```python
from build123d import *

# Parameters (mm, degrees)
SKETCH_1_R          = 3.75
SKETCH_1_R_2        = 2.75
EXTRUDE_436_DEPTH   = 4
EXTRUDE_START       = 4
SKETCH_2_R          = 1.7
SKETCH_2_R_2        = 2.75
EXTRUDE_712_DEPTH   = 5
SKETCH_3_R          = 2.9
EXTRUDE_5_8_DEPTH   = 9
SKETCH_4_R          = 2.9
EXTRUDE_5_8_2_DEPTH = 9


with BuildPart() as part:
    # 草图1 → Extrude 436 (new body)
    with BuildSketch(Plane.XY):
        Polygon((-44.899888641, -10), (-44.2082264, -12.713485699), (-43.352738806, -15.379858192), (-42.336596099, -17.989236526), (-41.163563864, -20.531950955), (-39.837989085, -22.998578775), (-38.364784033, -25.379979238), (-36.74940806, -27.667327432), (-34.997847373, -29.852146979), (-33.116592846, -31.926341448), (-31.112615968, -33.882224361), (-28.993343009, -35.712547671), (-26.7666275, -37.410528629), (-24.440721127, -38.969874914), (-22.024243155, -40.384807953), (-19.526148488, -41.650084336), (-16.955694479, -42.761015244), (-14.322406631, -43.713483827), (-11.636043292, -44.503960459), (-8.906559497, -45.129515818), (-6.144070075, -45.587831742), (-3.358812166, -45.87720982), (-0.561107284, -45.996577684), (2.238676931, -45.945492985), (5.030165132, -45.72414503), (7.803012717, -45.333354084), (10.546944161, -44.774568327), (13.251791096, -44.049858487), (15.907529991, -43.161910171), (18.504319299, -42.114013906), (21.032535927, -40.910052952), (23.482810893, -39.554488905), (25.846064052, -38.052345171), (28.11353774, -36.409188342), (30.276829231, -34.631107573), (32.327921871, -32.724692016), (34.25921479, -30.697006401), (36.063551069, -28.555564857), (37.734244259, -26.308303066), (39.265103162, -23.963548854), (40.650454772, -21.529991333), (41.885165301, -19.016648698), (42.9646592, -16.432834808), (43.884936117, -13.788124675), (44.64258572, -11.092318975), (45.234800338, -8.355407734), (45.659385361, -5.587533306), (45.914767377, -2.798952785), (46, 0), (45.914767377, 2.798952785), (45.659385361, 5.587533306), (45.234800338, 8.355407734), (44.64258572, 11.092318975), (43.884936117, 13.788124675), (42.9646592, 16.432834808), (41.885165301, 19.016648698), (40.650454772, 21.529991333), (39.265103162, 23.963548854), (37.734244259, 26.308303066), (36.063551069, 28.555564857), (34.25921479, 30.697006401), (32.327921871, 32.724692016), (30.276829231, 34.631107573), (28.11353774, 36.409188342), (25.846064052, 38.052345171), (23.482810893, 39.554488905), (21.032535927, 40.910052952), (18.504319299, 42.114013906), (15.907529991, 43.161910171), (13.251791096, 44.049858487), (10.546944161, 44.774568327), (7.803012717, 45.333354084), (5.030165132, 45.72414503), (2.238676931, 45.945492985), (-0.561107284, 45.996577684), (-3.358812166, 45.87720982), (-6.144070075, 45.587831742), (-8.906559497, 45.129515818), (-11.636043292, 44.503960459), (-14.322406631, 43.713483827), (-16.955694479, 42.761015244), (-19.526148488, 41.650084336), (-22.024243155, 40.384807953), (-24.440721127, 38.969874914), (-26.7666275, 37.410528629), (-28.993343009, 35.712547671), (-31.112615968, 33.882224361), (-33.116592846, 31.926341448), (-34.997847373, 29.852146979), (-36.74940806, 27.667327432), (-38.364784033, 25.379979238), (-39.837989085, 22.998578775), (-41.163563864, 20.531950955), (-42.336596099, 17.989236526), (-43.352738806, 15.379858192), (-44.2082264, 12.713485699), (-44.899888641, 10), (12, 10), (12, -10), align=None)
        with Locations((-14.845, -14.845)):
            Circle(SKETCH_1_R, mode=Mode.SUBTRACT)
        with Locations((-14.845, 14.845)):
            Circle(SKETCH_1_R, mode=Mode.SUBTRACT)
        with Locations((14.845, -14.845)):
            Circle(SKETCH_1_R, mode=Mode.SUBTRACT)
        with Locations((14.845, 14.845)):
            Circle(SKETCH_1_R, mode=Mode.SUBTRACT)
        with Locations((0, -40.5)):
            Circle(SKETCH_1_R_2, mode=Mode.SUBTRACT)
        with Locations((0, 40.5)):
            Circle(SKETCH_1_R_2, mode=Mode.SUBTRACT)
        with Locations((40.5, 0)):
            Circle(SKETCH_1_R_2, mode=Mode.SUBTRACT)
    extrude(amount=EXTRUDE_436_DEPTH)

    # 草图2 → Extrude 712 (add)
    with BuildSketch(Plane.XY.offset(EXTRUDE_START)):
        Polygon((-44.899888641, -10), (-44.2082264, -12.713485699), (-43.352738806, -15.379858192), (-42.336596099, -17.989236526), (-41.163563864, -20.531950955), (-39.837989085, -22.998578775), (-38.364784033, -25.379979238), (-36.74940806, -27.667327432), (-34.997847373, -29.852146979), (-33.116592846, -31.926341448), (-31.112615968, -33.882224361), (-28.993343009, -35.712547671), (-26.7666275, -37.410528629), (-24.440721127, -38.969874914), (-22.024243155, -40.384807953), (-19.526148488, -41.650084336), (-16.955694479, -42.761015244), (-14.322406631, -43.713483827), (-11.636043292, -44.503960459), (-8.906559497, -45.129515818), (-6.144070075, -45.587831742), (-3.358812166, -45.87720982), (-0.561107284, -45.996577684), (2.238676931, -45.945492985), (5.030165132, -45.72414503), (7.803012717, -45.333354084), (10.546944161, -44.774568327), (13.251791096, -44.049858487), (15.907529991, -43.161910171), (18.504319299, -42.114013906), (21.032535927, -40.910052952), (23.482810893, -39.554488905), (25.846064052, -38.052345171), (28.11353774, -36.409188342), (30.276829231, -34.631107573), (32.327921871, -32.724692016), (34.25921479, -30.697006401), (36.063551069, -28.555564857), (37.734244259, -26.308303066), (39.265103162, -23.963548854), (40.650454772, -21.529991333), (41.885165301, -19.016648698), (42.9646592, -16.432834808), (43.884936117, -13.788124675), (44.64258572, -11.092318975), (45.234800338, -8.355407734), (45.659385361, -5.587533306), (45.914767377, -2.798952785), (46, 0), (45.914767377, 2.798952785), (45.659385361, 5.587533306), (45.234800338, 8.355407734), (44.64258572, 11.092318975), (43.884936117, 13.788124675), (42.9646592, 16.432834808), (41.885165301, 19.016648698), (40.650454772, 21.529991333), (39.265103162, 23.963548854), (37.734244259, 26.308303066), (36.063551069, 28.555564857), (34.25921479, 30.697006401), (32.327921871, 32.724692016), (30.276829231, 34.631107573), (28.11353774, 36.409188342), (25.846064052, 38.052345171), (23.482810893, 39.554488905), (21.032535927, 40.910052952), (18.504319299, 42.114013906), (15.907529991, 43.161910171), (13.251791096, 44.049858487), (10.546944161, 44.774568327), (7.803012717, 45.333354084), (5.030165132, 45.72414503), (2.238676931, 45.945492985), (-0.561107284, 45.996577684), (-3.358812166, 45.87720982), (-6.144070075, 45.587831742), (-8.906559497, 45.129515818), (-11.636043292, 44.503960459), (-14.322406631, 43.713483827), (-16.955694479, 42.761015244), (-19.526148488, 41.650084336), (-22.024243155, 40.384807953), (-24.440721127, 38.969874914), (-26.7666275, 37.410528629), (-28.993343009, 35.712547671), (-31.112615968, 33.882224361), (-33.116592846, 31.926341448), (-34.997847373, 29.852146979), (-36.74940806, 27.667327432), (-38.364784033, 25.379979238), (-39.837989085, 22.998578775), (-41.163563864, 20.531950955), (-42.336596099, 17.989236526), (-43.352738806, 15.379858192), (-44.2082264, 12.713485699), (-44.899888641, 10), (12, 10), (12, -10), align=None)
        with Locations((-14.845, -14.845)):
            Circle(SKETCH_2_R, mode=Mode.SUBTRACT)
        with Locations((-14.845, 14.845)):
            Circle(SKETCH_2_R, mode=Mode.SUBTRACT)
        with Locations((14.845, -14.845)):
            Circle(SKETCH_2_R, mode=Mode.SUBTRACT)
        with Locations((14.845, 14.845)):
            Circle(SKETCH_2_R, mode=Mode.SUBTRACT)
        with Locations((0, -40.5)):
            Circle(SKETCH_2_R_2, mode=Mode.SUBTRACT)
        with Locations((0, 40.5)):
            Circle(SKETCH_2_R_2, mode=Mode.SUBTRACT)
        with Locations((40.5, 0)):
            Circle(SKETCH_2_R_2, mode=Mode.SUBTRACT)
    extrude(amount=EXTRUDE_712_DEPTH)

    # 草图3 → Extrude 5.8 (add)
    with BuildSketch(Plane.XY):
        with BuildLine():
            Line((-33.234018716, -14.849242405), (-69.028961031, -56.301038969))
            ThreePointArc((-69.028961031, -56.301038969), (-69.028961031, -69.028961031), (-56.301038969, -69.028961031))
            Line((-56.301038969, -69.028961031), (-14.849242405, -33.234018716))
            Line((-14.849242405, -33.234018716), (-33.234018716, -14.849242405))
        make_face()
        with Locations((-62.665, -62.665)):
            Circle(SKETCH_3_R, mode=Mode.SUBTRACT)
    extrude(amount=EXTRUDE_5_8_DEPTH)

    # 草图4 → Extrude 5.8 2 (add)
    with BuildSketch(Plane.XY):
        with BuildLine():
            Line((-14.849242405, 33.234018716), (-56.301038969, 69.028961031))
            ThreePointArc((-56.301038969, 69.028961031), (-69.028961031, 69.028961031), (-69.028961031, 56.301038969))
            Line((-69.028961031, 56.301038969), (-33.234018716, 14.849242405))
            Line((-33.234018716, 14.849242405), (-14.849242405, 33.234018716))
        make_face()
        with Locations((-62.665, 62.665)):
            Circle(SKETCH_4_R, mode=Mode.SUBTRACT)
    extrude(amount=EXTRUDE_5_8_2_DEPTH)


solid = part.part
```
Check sheet for the modelled part. Datum: model origin and axes. Units: mm. A direction names the side the tool comes from. Give positions to 0.01 mm unless a question says otherwise; leave off trailing zeros. Order: outer loops, then holes, each group sorted by start corner. A loop starts at its lowest first (then second) coordinate and runs counter-clockwise, first axis right, second up. Notation, with made-up numbers: M 54.25,-31.5 L 60.25,-31.5 A23 ccw 60.25,-22.5 Z; hole C 84,2 d2. An arc over 180 degrees is marked long. Answer in a Markdown table with one row per item. Add a question column.
Q1. Release check for a two-part mould opening along X. For faces 1 (the flat face through (13, -15, 4)), 2 (the cylindrical face through (-68.887, 69.167, 4.437)), 3 (the flat face through (45.79, 4.17, 4.44)), 4 (the flat face through (16, 13, 4)) record: released by +X, released by -X, zero draft, split by the parting line, or undercut.
Q2. Gauge pin test, flat ends, axial feed: pin 1 Ø4.5 at (x, y) = (-14.845, -14.845) entering from -Z; pin 2 Ø3 at (y, z) = (50, 5.5) entering from +X; pin 3 Ø4.5 at (x, y) = (-62.665, -62.665) entering from -Z; pin 4 Ø4.5 at (x, y) = (14.845, 14.845) entering from +Z. Record the tip position at first contact, or that the pin passes through.
Q3. Thickness scan on L1, parallel to Y at x = 6, z = 4; L2, parallel to Y at x = 0, z = 4.75; L3, parallel to X at y = 15.5, z = 1.5. Record the ranges inside material, lowest first.
Q4. Sectioned sample at A-A, the plane x = -49. Record the boundary of the cut face in (y, z), and give its area (3 significant figures).
Q5. Sectioned sample at C-C, the plane z = 2. Count the separate pieces of the cut face and the enclosed holes in it, and give its area (3 significant figures).
Q6. Sectioned sample at B-B, the plane x = -33.5. Record the boundary of the cut face in (y, z).
Q7. Access from +Z, -Z, +X, -X, +Y, -Y to the whole of each face (thin tool, end or side, straight path). Record for faces 5 (the cylindrical face through (14.032, 11.184, 1.972)), 6 (the flat face through (-1.98, -45.936, 4.437)), 7 (the flat face through (-54.313, -39.26, 4.437)).
Verdict:
| question | item | result |
|---|---|---|
| 1 | face 1 | undercut |
| 1 | face 2 | split by the parting line |
| 1 | face 3 | released by +X |
| 1 | face 4 | undercut |
| 2 | pin 1 | z = 4 |
| 2 | pin 2 | x = -32.53 |
| 2 | pin 3 | through |
| 2 | pin 4 | z = 9 |
| 3 | L1 | -45.59 to -10, 10 to 45.59 |
| 3 | L2 | -45.99 to -43.25, -37.75 to -10, 10 to 37.75, 43.25 to 45.99 |
| 3 | L3 | -43.31 to -18.54, -11.15 to 11.15, 18.54 to 43.29 |
| 4 | outline | M -62.72,0 L -33.11,0 L -33.11,9 L -62.72,9 Z; M 33.11,0 L 62.72,0 L 62.72,9 L 33.11,9 Z |
| 4 | area | 533 mm² |
| 5 | separate pieces | 1 |
| 5 | enclosed holes | 9 |
| 5 | area | 7,270 mm² |
| 6 | outline | M -49.34,0 L -10,0 L -10,9 L -49.34,9 Z; M 10,0 L 49.34,0 L 49.34,9 L 10,9 Z |
| 7 | face 5 | -Z |
| 7 | face 6 | +Z, -Z, -Y |
| 7 | face 7 | +Z, -Z, -X |
